from build123d import *

# Parameters (mm, degrees)
F0_W     = 15
F0_H     = 2.75
F0_H_2   = 5.2
F0_R     = 1.9
F0_H_3   = 4.3
F1_DEPTH = 3
F2_DEPTH = 1.3
F3_R     = 4.99999


# Not quite as in the source:
# - a fillet or chamfer is up to 0.001 mm smaller than in the source, because OpenCascade refuses the exact size
# - a feature names something its author has since deleted; it is built from what else it names


with BuildPart() as f1:
    # F0 (on Top) → F1 (new body)
    with BuildSketch(Plane.XY):
        with Locations((0, 8.825)):
            Rectangle(F0_W, F0_H)
        with Locations((0, 12.8)):
            Rectangle(F0_W, F0_H_2)
        with Locations((0, 12.8)):
            Circle(F0_R, mode=Mode.SUBTRACT)
        with Locations((0, 17.55)):
            Rectangle(F0_W, F0_H_3)
        Polygon((-7.5, 27.2), (-7.5, 19.7), (7.5, 19.7), (12.5, 19.7), (12.5, 34.7), (5, 27.2), align=None)
    extrude(amount=F1_DEPTH)

    # F0 (on Top) → F2 (join)
    with BuildSketch(Plane.XY):
        with Locations((0, 12.8)):
            Rectangle(F0_W, F0_H_2)
        with Locations((0, 12.8)):
            Circle(F0_R, mode=Mode.SUBTRACT)
    extrude(amount=-F2_DEPTH)

    # F3 (radius 5 in the source; OpenCascade refuses exactly that, so slightly less here)
    f3_edges = [f1.edges().sort_by_distance(p)[0] for p in [
        (12.5, 19.7, 1.5),
        (-7.5, 27.2, 1.5),
        (5, 27.2, 1.5),
    ]]
    fillet(f3_edges, radius=F3_R)


solid = f1.part
Can you work these out from the model? Positions are in its coordinate system, mm. A direction names the side the tool comes from. Coordinates: 2 decimals unless noted, no trailing zeros. Loops run counter-clockwise (first coordinate to the right, second up) from the corner with the lowest first, then second, coordinate; pieces in that order, holes last. Notation, with made-up numbers: (14, 41) - (28, 41) arc R14 ccw to (28, 56) - close; hole circle Ø8 at (67.25, 61.5). An arc over 180 degrees is marked (long way). Answer as a JSON object with one key per item and string values. Group by question number.
Item 1: If I drill on L1, parallel to Y at x = 0, z = 1.95; L2, parallel to X at y = 15, z = 0.1; L3, parallel to Z at x = 6, y = 15.5, over which ranges is the centre line in solid material (lowest first)? Write a range as from..to.
Item 2: If we section it at D-D (x = 7): List the corners of the cut face in (y, z) for me.
Item 3: If we section it at A-A (y = 12.8): List the corners of the cut face in (x, z) for me.
Item 4: If we mould it in two halves opening along X, with no side actions, what happens to faces 1 (the face through (-6.07, 25.7, 1.52)), 2 (the face through (0, 9, 0)), 3 (the face through (0.877, 11.114, 0.82))? For each: released by +X, released by -X, zero draft, split by the parting line, or undercut.
Item 5: If we section it at B-B (x = 0): List the corners of the cut face in (y, z) for me, plus the area to 3 significant figures.
Item 6: On a 3-axis mill with a long thin cutter (end or side, diameter ignored), from which of +Z, -Z, +X, -X, +Y, -Y can I reach the whole of each face in a straight line? I mean faces 4 (the face through (7.5, 13, 1)), 5 (the face through (0, 27.2, 1)), 6 (the face through (0, 10.2, -1)). Say none if no direction works.
Item 7: For pin 1 (2 mm diameter, centred on y = 14.5, z = 0, fed in from +X); pin 2 (9.5 mm diameter, centred on x = 2.5, y = 25, fed in from -Z); pin 3 (1.5 mm diameter, centred on x = 9.5, z = -0.5, fed in from -Y); pin 4 (6 mm diameter, centred on x = 0, y = 12.8, fed in from +Z), each with a flat end and sliding along its axis, tell me the tip position at first contact or that it passes through.
Returned:
{
 "1": {"L1": "y = 7.45..10.9, 14.7..27.2", "L2": "x = -7.5..7.5", "L3": "z = 0..3"},
 "2": {"outline": "(7.45, 0) - (10.2, 0) - (10.2, -1.3) - (15.4, -1.3) - (15.4, 0) - (29.2, 0) - (29.2, 3) - (7.45, 3) - close"},
 "3": {"outline": "(-7.5, -1.3) - (-1.9, -1.3) - (-1.9, 3) - (-7.5, 3) - close; (1.9, -1.3) - (7.5, -1.3) - (7.5, 3) - (1.9, 3) - close"},
 "4": {"face 1": "released by -X", "face 2": "zero draft", "face 3": "undercut"},
 "5": {"outline": "(7.45, 0) - (10.2, 0) - (10.2, -1.3) - (10.9, -1.3) - (10.9, 3) - (7.45, 3) - close; (14.7, -1.3) - (15.4, -1.3) - (15.4, 0) - (27.2, 0) - (27.2, 3) - (14.7, 3) - close", "area": "49.7 mm²"},
 "6": {"face 4": "+Z, -Z, +X, -Y", "face 5": "+Z, -Z, -X, +Y", "face 6": "-Z, +X, -X, -Y"},
 "7": {"pin 1": "stops at x = 7.5", "pin 2": "stops at z = 0", "pin 3": "stops at y = 19.91", "pin 4": "stops at z = 3"}
}
